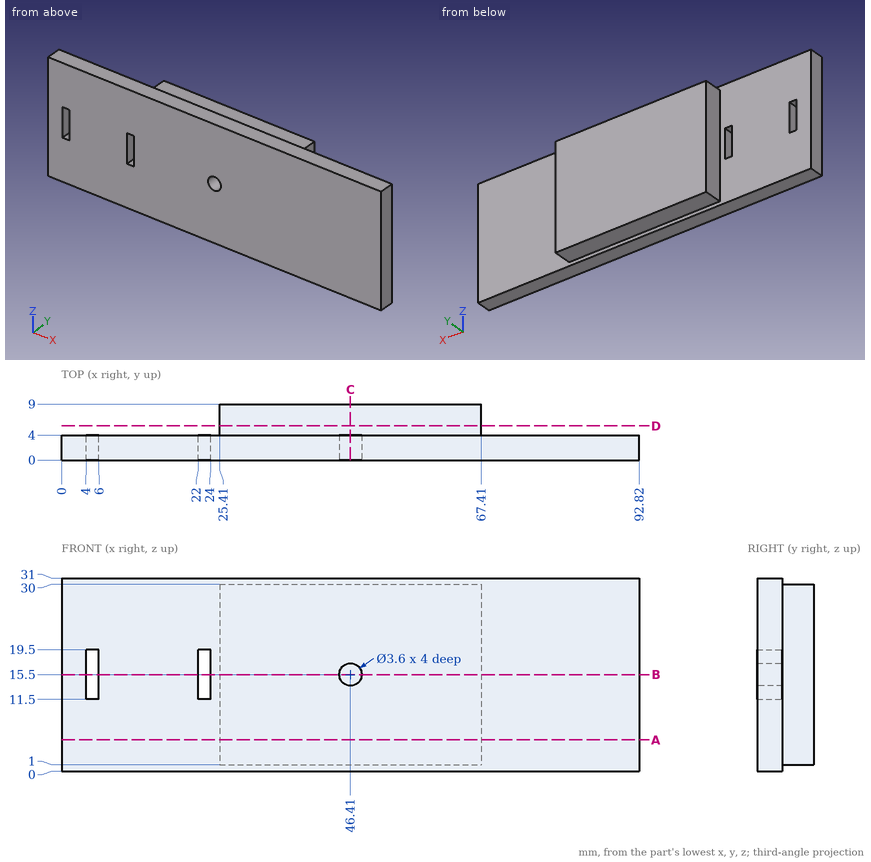
Geometry check sheet. Reference: drawing and pictorial views, mm from the part's lowest x, y, z. Give positions to 0.01 mm unless a question says otherwise; leave off trailing zeros. Write each loop counter-clockwise with the first axis right and the second up, starting at its lowest first coordinate (ties: lowest second). Pieces come first, ordered by that corner, then holes. Notation, with made-up numbers: M 15,24 L 30,24 A20 ccw 30,36 Z; hole C -5.75,78.25 d10. An arc over 180 degrees is marked long. Put each result on its own line as item: value. Start each with the question number.
1. Scan lines: line 1 along X through (y, z) = (2, 15.5); line 2 along X through (y, z) = (2.5, 14.5); line 3 along X through (y, z) = (5, 8.5). Record each from-to range of solid material in increasing order. Write a range as [from, to].
2. Section check C-C (x = 46.41). Record the cut outline in (y, z).
3. Go/stop test with flat-tipped pins: pin 1 Ø1.5 at (y, z) = (5.5, 28) entering from -X; pin 2 Ø1.5 at (x, y) = (41.5, 7.5) entering from -Z; pin 3 Ø5 at (x, z) = (70, 19) entering from +Y. Record where each tip stops, or that it passes through.
4. Section check D-D (y = 5.5). Record the cut outline in (x, z), and give its area (3 significant figures).
5. Section check A-A (z = 5). Record the cut outline in (x, y), and give its area (3 significant figures).
6. Section check B-B (z = 15.5). Record the cut outline in (x, y), and give its area (3 significant figures).
Answer list:
1. line 1: [0, 4], [6, 22], [24, 44.61], [48.21, 92.82]
1. line 2: [0, 4], [6, 22], [24, 44.91], [47.91, 92.82]
1. line 3: [25.41, 67.41]
2. outline: M 0,0 L 4,0 L 4,1 L 9,1 L 9,30 L 4,30 L 4,31 L 0,31 L 0,17.3 L 4,17.3 L 4,13.7 L 0,13.7 Z
3. pin 1: x = 25.41
3. pin 2: z = 1
3. pin 3: y = 4
4. outline: M 25.41,1 L 67.41,1 L 67.41,30 L 25.41,30 Z
4. area: 1,220 mm2
5. outline: M 0,0 L 92.82,0 L 92.82,4 L 67.41,4 L 67.41,9 L 25.41,9 L 25.41,4 L 0,4 Z
5. area: 581 mm2
6. outline: M 0,0 L 4,0 L 4,4 L 0,4 Z; M 6,0 L 22,0 L 22,4 L 6,4 Z; M 24,0 L 44.61,0 L 44.61,4 L 48.21,4 L 48.21,0 L 92.82,0 L 92.82,4 L 67.41,4 L 67.41,9 L 25.41,9 L 25.41,4 L 24,4 Z
6. area: 551 mm2
